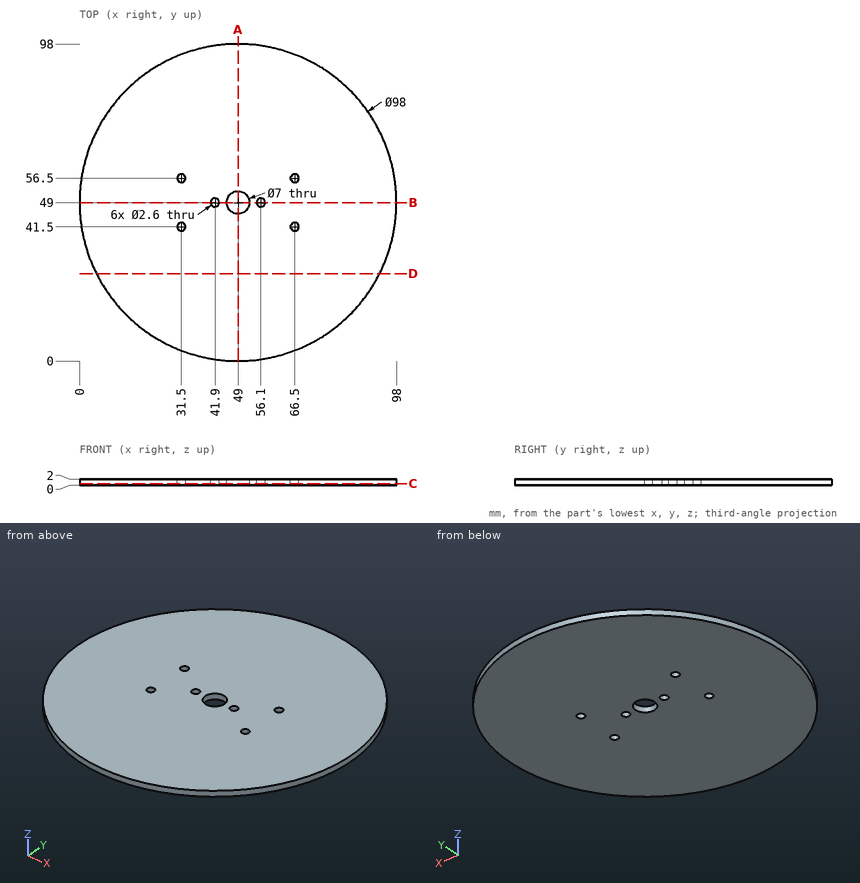
The drawing under review shows one solid part. Ordinate dimensions are in mm from its lowest x, y, z. Round coordinates to 2 decimals unless told otherwise and drop trailing zeros. Loops run counter-clockwise (first coordinate to the right, second up) from the corner with the lowest first, then second, coordinate; pieces in that order, holes last. Notation, with made-up numbers: (26, 69.25) - (60, 69.25) arc R19 ccw to (60, 104.25) - close; hole circle Ø7 at (-9, 62). An arc over 180 degrees is marked (long way). One line per item, written item: value. Start each with the question number.
1) Consider section A-A on x = 49. Give the boundary of the cut face in (y, z), then the cut area to 3 significant figures.
2) To check wall thickness, follow L1, parallel to Y at x = 31.5, z = 1.55; L2, parallel to Y at x = 49, z = 1.5; L3, parallel to Y at x = 55, z = 0.9. State the ranges of each line that lie inside material, in increasing order. Write a range as from..to.
3) Insertion check: pin 1 Ø1 at (x, z) = (21.5, 1) entering from +Y. The pin has a flat end and moves straight along its axis. Give the tip position at first contact, or say it passes through.
4) Consider section B-B on y = 49. Give the boundary of the cut face in (x, z), then the cut area to 3 significant figures.
5) Consider section C-C on z = 0.6. Give the boundary of the cut face in (x, y), then the cut area to 3 significant figures.
6) Consider section D-D on y = 27. Give the boundary of the cut face in (x, z), then the cut area to 3 significant figures.
Reported:
1. outline: (0, 0) - (45.5, 0) - (45.5, 2) - (0, 2) - close; (52.5, 0) - (98, 0) - (98, 2) - (52.5, 2) - close
1. area: 182 mm^2
2. L1: y = 3.23..40.2, 42.8..55.2, 57.8..94.77
2. L2: y = 0..45.5, 52.5..98
2. L3: y = 0.37..48.31, 49.69..97.63
3. pin 1: stops at y = 89.89
4. outline: (0, 0) - (40.6, 0) - (40.6, 2) - (0, 2) - close; (43.2, 0) - (45.5, 0) - (45.5, 2) - (43.2, 2) - close; (52.5, 0) - (54.8, 0) - (54.8, 2) - (52.5, 2) - close; (57.4, 0) - (98, 0) - (98, 2) - (57.4, 2) - close
4. area: 172 mm^2
5. outline: circle Ø98 at (49, 49); hole circle Ø2.6 at (31.5, 41.5); hole circle Ø2.6 at (31.5, 56.5); hole circle Ø2.6 at (41.9, 49); hole circle Ø7 at (49, 49); hole circle Ø2.6 at (56.1, 49); hole circle Ø2.6 at (66.5, 41.5); hole circle Ø2.6 at (66.5, 56.5)
5. area: 7,470 mm^2
6. outline: (5.22, 0) - (92.78, 0) - (92.78, 2) - (5.22, 2) - close
6. area: 175 mm^2
